from build123d import *

# Parameters (mm, degrees)
SKETCH1_W           = 43.18
SKETCH1_H           = 17.78
SKETCH1_R           = 1.27
BOSS_EXTRUDE1_DEPTH = 1.2
FILLET1_R           = 2.54
SKETCH2_W           = 5
SKETCH2_H           = 7
BOSS_EXTRUDE2_DEPTH = 3


with BuildPart() as part:
    # Sketch1 → Boss-Extrude1 (new body)
    with BuildSketch(Plane(origin=(0, 0, 0), x_dir=(1, 0, 0), z_dir=(0, 1, 0))):
        with Locations((-21.59, 8.89)):
            Rectangle(SKETCH1_W, SKETCH1_H)
        with Locations(Location((-40.64, 15.24, 0), (0, 0, 270))):
            Circle(SKETCH1_R, mode=Mode.SUBTRACT)
        with Locations(Location((-40.64, 2.54, 0), (0, 0, 270))):
            Circle(SKETCH1_R, mode=Mode.SUBTRACT)
        with Locations(Location((-2.54, 2.54, 0), (0, 0, 270))):
            Circle(SKETCH1_R, mode=Mode.SUBTRACT)
        with Locations(Location((-2.54, 15.24, 0), (0, 0, 270))):
            Circle(SKETCH1_R, mode=Mode.SUBTRACT)
    extrude(amount=BOSS_EXTRUDE1_DEPTH)

    # Fillet1
    fillet1_edges = [part.edges().sort_by_distance(p)[0] for p in [
        (0, 0.6, 0),
        (-43.18, 0.6, 0),
        (-43.18, 0.6, -17.78),
        (0, 0.6, -17.78),
    ]]
    fillet(fillet1_edges, radius=FILLET1_R)

    # Sketch2 → Boss-Extrude2 (add)
    with BuildSketch(Plane(origin=(0, 1.2, 0), x_dir=(1, 0, 0), z_dir=(0, 1, 0))):
        with Locations((-40.68, 8.89)):
            Rectangle(SKETCH2_W, SKETCH2_H)
    extrude(amount=BOSS_EXTRUDE2_DEPTH)


solid = part.part
Here's how the part is built. I have some questions about the finished solid (model axes, mm). A direction names the side the tool comes from. Give positions to 0.01 mm unless a question says otherwise; leave off trailing zeros. Order: outer loops, then holes, each group sorted by start corner. A loop starts at its lowest first (then second) coordinate and runs counter-clockwise, first axis right, second up. Notation, with made-up numbers: M 78,32.5 L 95,32.5 A27 cw 95,51.5 Z; hole C -23,52.5 d3. An arc over 180 degrees is marked long. Answer as a JSON object with one key per item and string values. Group by question number.
1) Please list where these lines run through material, in increasing order: L1, parallel to X at y = 0.5, z = -15.24; L2, parallel to Y at x = -22.5, z = -7.5; L3, parallel to Z at x = -3.5, y = 0.8. Write a range as [from, to].
2) Suppose I cut it at B-B, the plane z = -8. Write out the boundary of the cut face in (x, y), plus the area to 3 significant figures.
3) On a 3-axis mill with a long thin cutter (end or side, diameter ignored), from which of +Z, -Z, +X, -X, +Y, -Y can I reach the whole of each face in a straight line? I mean faces 4 (the cylindrical face through (-42.456, 0.608, -17.016)), 5 (the flat face through (-41, 3, -5.39)), 6 (the flat face through (-41, 3, -12.39)), 7 (the flat face through (-38.18, 3, -9)). Say none if no direction works.
4) We'd pull the mould along Z, two halves only. Please class faces 1 (the cylindrical face through (-0.764, 0.608, -0.724)), 2 (the flat face through (-43.18, 2, -9)), 3 (the cylindrical face through (-40.58, 0.59, -16.51)): pulls with the +Z half, pulls with the -Z half, needs draft (parallel to the pull), parting line crosses it, or undercut.
5) Suppose I cut it at C-C, the plane x = -13.5. Write out the boundary of the cut face in (y, z), plus the area to 3 significant figures.
6) Suppose I cut it at A-A, the plane y = 0.5. Write out the boundary of the cut face in (x, z).
7) I'm going to push flat-ended pins straight in: pin 1 Ø0.9 at (x, y) = (-41.5, 2.5) entering from +Z; pin 2 Ø1.5 at (x, y) = (-41, 3) entering from -Z; pin 3 Ø4 at (x, z) = (-40.64, -2.54) entering from +Y; pin 4 Ø2 at (x, z) = (-2.54, -15.24) entering from -Y. Where does each tip first touch, or does it pass through?
Results found:
{
 "1": {"L1": "[-43.18, -41.91], [-39.37, -3.81], [-1.27, 0]", "L2": "[0, 1.2]", "L3": "[-17.78, -16.07], [-14.41, -3.37], [-1.71, 0]"},
 "2": {"outline": "M -43.18,0 L 0,0 L 0,1.2 L -38.18,1.2 L -38.18,4.2 L -43.18,4.2 Z", "area": "66.8 mm²"},
 "3": {"face 4": "-Z, -X, +Y, -Y", "face 5": "+Z, +X, -X, +Y", "face 6": "-Z, +X, -X, +Y", "face 7": "+Z, -Z, +X, +Y"},
 "4": {"face 1": "pulls with the +Z half", "face 2": "needs draft", "face 3": "undercut"},
 "5": {"outline": "M 0,-17.78 L 1.2,-17.78 L 1.2,0 L 0,0 Z", "area": "21.3 mm²"},
 "6": {"outline": "M -43.18,-15.24 A2.54 ccw -40.64,-17.78 L -2.54,-17.78 A2.54 ccw 0,-15.24 L 0,-2.54 A2.54 ccw -2.54,0 L -40.64,0 A2.54 ccw -43.18,-2.54 Z; hole C -40.64,-15.24 d2.54; hole C -40.64,-2.54 d2.54; hole C -2.54,-15.24 d2.54; hole C -2.54,-2.54 d2.54"},
 "7": {"pin 1": "z = -5.39", "pin 2": "z = -12.39", "pin 3": "y = 1.2", "pin 4": "through"}
}
